Verification items for this drawing (mm, ordinates from the low corner). A direction names the side the tool comes from. Give positions to 0.01 mm unless a question says otherwise; leave off trailing zeros. Order: outer loops, then holes, each group sorted by start corner. A loop starts at its lowest first (then second) coordinate and runs counter-clockwise, first axis right, second up. Notation, with made-up numbers: M 40,-24 L 83,-24 A21 ccw 83,-16 Z; hole C -39,59 d5. An arc over 180 degrees is marked long. Return JSON: item names as keys, results as strings. Group by question number.
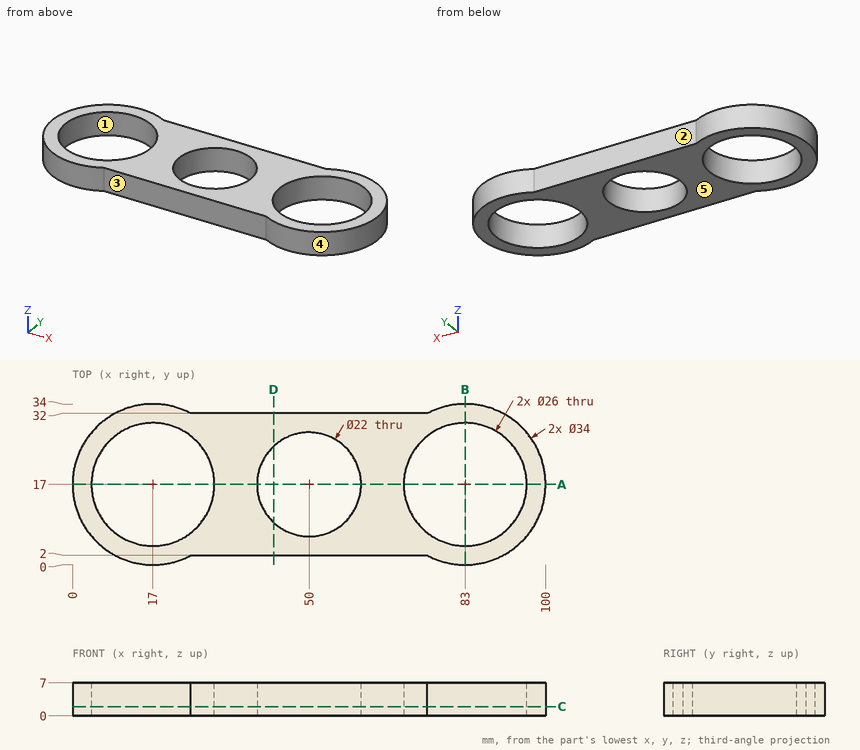
1) Tool access check on the marked faces 1, 2 and 3. Record the directions out of +Z, -Z, +X, -X, +Y, -Y that give a thin tool (end or side, any length) a straight path to the whole face; none if there is none.
2) Sectioned sample at B-B on x = 83. Record the boundary of the cut face in (y, z).
3) Sectioned sample at C-C on z = 2. Record the boundary of the cut face in (x, y), then the cut area to 3 significant figures.
4) Release check for a two-part mould opening along X. For the marked faces 4 and 5 record: released by +X, released by -X, zero draft, split by the parting line, or undercut.
5) Sectioned sample at A-A on y = 17. Record the boundary of the cut face in (x, z), then the cut area to 3 significant figures.
6) Material ranges on line 1 along Y through (x, z) = (50, 3.5); line 2 along Y through (x, z) = (83, 4.25); line 3 along X through (y, z) = (29, 2.5), recorded low to high.
7) Depth check by flat-ended pin: P1, Ø2, axis at x = 49.5, z = 2.5, coming from the +Y side; P2, Ø2, axis at y = 10.5, z = 1, coming from the -X side; P3, Ø2, axis at y = 25, z = 2.5, coming from the -X side. Enter the tip coordinate at first touch or a pass-through.
8) Sectioned sample at D-D on x = 42.5. Record the boundary of the cut face in (y, z).
Reply:
{
 "1": {"face 1": "+Z, -Z", "face 2": "+Z, -Z, +Y", "face 3": "+Z, -Z, -Y"},
 "2": {"outline": "M 0,0 L 4,0 L 4,7 L 0,7 Z; M 30,0 L 34,0 L 34,7 L 30,7 Z"},
 "3": {"outline": "M 25,2 L 75,2 A17 ccw long 75,32 L 25,32 A17 ccw long Z; hole C 17,17 d26; hole C 50,17 d22; hole C 83,17 d26", "area": "1,490 mm^2"},
 "4": {"face 4": "undercut", "face 5": "zero draft"},
 "5": {"outline": "M 0,0 L 4,0 L 4,7 L 0,7 Z; M 30,0 L 39,0 L 39,7 L 30,7 Z; M 61,0 L 70,0 L 70,7 L 61,7 Z; M 96,0 L 100,0 L 100,7 L 96,7 Z", "area": "182 mm^2"},
 "6": {"line 1": "2 to 6, 28 to 32", "line 2": "0 to 4, 30 to 34", "line 3": "4.96 to 12, 22 to 78, 88 to 95.04"},
 "7": {"P1": "y = 32", "P2": "x = 0.91", "P3": "x = 1.51"},
 "8": {"outline": "M 2,0 L 8.95,0 L 8.95,7 L 2,7 Z; M 25.05,0 L 32,0 L 32,7 L 25.05,7 Z"}
}
